Could you check a few things on this model? Use its own coordinates, in mm. A direction names the side the tool comes from. Round coordinates to 2 decimals unless told otherwise and drop trailing zeros. Loops run counter-clockwise (first coordinate to the right, second up) from the corner with the lowest first, then second, coordinate; pieces in that order, holes last.
from build123d import *

# Parameters (mm, degrees)
F2_R     = 7.5
F2_R_2   = 5.5
F3_DEPTH = 3
F4_DEPTH = 5


# Not quite as in the source:
# - a feature names something its author has since deleted; it is built from what else it names


with BuildPart() as f3:
    # F2 (on Top) → F3 (new body)
    with BuildSketch(Plane.XY):
        with BuildLine():
            Line((120, 9.5), (0, 9.5))
            ThreePointArc((0, 9.5), (-6.7175144213, 6.7175144213), (-9.5, 0))
            ThreePointArc((-9.5, 0), (-6.7175144213, -6.7175144213), (0, -9.5))
            Line((0, -9.5), (120, -9.5))
            ThreePointArc((120, -9.5), (126.7175144213, -6.7175144213), (129.5, 0))
            ThreePointArc((129.5, 0), (126.7175144213, 6.7175144213), (120, 9.5))
        make_face()
        Circle(F2_R, mode=Mode.SUBTRACT)
        with Locations((20, 0)):
            Circle(F2_R, mode=Mode.SUBTRACT)
        with Locations((40, 0)):
            Circle(F2_R, mode=Mode.SUBTRACT)
        with Locations((60, 0)):
            Circle(F2_R, mode=Mode.SUBTRACT)
        with Locations((80, 0)):
            Circle(F2_R, mode=Mode.SUBTRACT)
        with Locations((100, 0)):
            Circle(F2_R, mode=Mode.SUBTRACT)
        with Locations((120, 0)):
            Circle(F2_R, mode=Mode.SUBTRACT)
        Circle(F2_R)
        Circle(F2_R_2, mode=Mode.SUBTRACT)
        with Locations((20, 0)):
            Circle(F2_R)
        with Locations((20, 0)):
            Circle(F2_R_2, mode=Mode.SUBTRACT)
        with Locations((40, 0)):
            Circle(F2_R)
        with Locations((40, 0)):
            Circle(F2_R_2, mode=Mode.SUBTRACT)
        with Locations((60, 0)):
            Circle(F2_R)
        with Locations((60, 0)):
            Circle(F2_R_2, mode=Mode.SUBTRACT)
        with Locations((80, 0)):
            Circle(F2_R)
        with Locations((80, 0)):
            Circle(F2_R_2, mode=Mode.SUBTRACT)
        with Locations((100, 0)):
            Circle(F2_R)
        with Locations((100, 0)):
            Circle(F2_R_2, mode=Mode.SUBTRACT)
        with Locations((120, 0)):
            Circle(F2_R)
        with Locations((120, 0)):
            Circle(F2_R_2, mode=Mode.SUBTRACT)
    extrude(amount=F3_DEPTH)

    # F2 (on Top) → F4 (join)
    with BuildSketch(Plane.XY):
        Circle(F2_R)
        Circle(F2_R_2, mode=Mode.SUBTRACT)
        with Locations((20, 0)):
            Circle(F2_R)
        with Locations((20, 0)):
            Circle(F2_R_2, mode=Mode.SUBTRACT)
        with Locations((40, 0)):
            Circle(F2_R)
        with Locations((40, 0)):
            Circle(F2_R_2, mode=Mode.SUBTRACT)
        with Locations((60, 0)):
            Circle(F2_R)
        with Locations((60, 0)):
            Circle(F2_R_2, mode=Mode.SUBTRACT)
        with Locations((80, 0)):
            Circle(F2_R)
        with Locations((80, 0)):
            Circle(F2_R_2, mode=Mode.SUBTRACT)
        with Locations((100, 0)):
            Circle(F2_R)
        with Locations((100, 0)):
            Circle(F2_R_2, mode=Mode.SUBTRACT)
        with Locations((120, 0)):
            Circle(F2_R)
        with Locations((120, 0)):
            Circle(F2_R_2, mode=Mode.SUBTRACT)
    extrude(amount=F4_DEPTH)


solid = f3.part
Item 1: We'd pull the mould along X, two halves only. Please class faces 3 (the cylindrical face through (12.507, 0.33, 3.986)), 4 (the flat face through (76, 4, 5)): released by +X, released by -X, zero draft, split by the parting line, or undercut.
Results list:
face 3: undercut
face 4: zero draft
Item 2: If I drill on line 1 along Y through (x, z) = (40, 2.4); line 2 along Z through (x, y) = (117.5, -7.75); line 3 along Y through (x, z) = (44.5, 2.75), over which ranges is the centre line in solid material (lowest first)?
Results list:
line 1: y = -9.5 to -5.5, 5.5 to 9.5
line 2: z = 0 to 3
line 3: y = -9.5 to -3.16, 3.16 to 9.5
Item 3: If we section it at A-A, the plane x = 80: Please give me the cut outline in (y, z).
Results list:
outline: (-9.5, 0) - (-5.5, 0) - (-5.5, 5) - (-7.5, 5) - (-7.5, 3) - (-9.5, 3) - close; (5.5, 0) - (9.5, 0) - (9.5, 3) - (7.5, 3) - (7.5, 5) - (5.5, 5) - close
Item 4: If we section it at C-C, the plane x = 104: Please give me the cut outline in (y, z), then the cut area to 3 significant figures.
Results list:
outline: (-9.5, 0) - (-3.77, 0) - (-3.77, 5) - (-6.34, 5) - (-6.34, 3) - (-9.5, 3) - close; (3.77, 0) - (9.5, 0) - (9.5, 3) - (6.34, 3) - (6.34, 5) - (3.77, 5) - close
area: 44.6 mm2
Item 5: If we section it at B-B, the plane z = 2: Please give me the cut outline in (x, y), then the cut area to 3 significant figures.
Results list:
outline: (0, -9.5) - (120, -9.5) arc R9.5 ccw to (120, 9.5) - (0, 9.5) arc R9.5 ccw to start; hole circle Ø11 at (0, 0); hole circle Ø11 at (20, 0); hole circle Ø11 at (40, 0); hole circle Ø11 at (60, 0); hole circle Ø11 at (80, 0); hole circle Ø11 at (100, 0); hole circle Ø11 at (120, 0)
area: 1,900 mm2
Item 6: If we section it at D-D, the plane y = 1.25: Count the separate pieces of the cut face and the enclosed holes in it, then the cut area to 3 significant figures.
Results list:
separate pieces: 8
enclosed holes: 0
area: 249 mm2
Item 7: For faces 1 (the flat face through (16, 4, 5)), 2 (the flat face through (59, -8, 3)), which set-ups out of +Z, -Z, +X, -X, +Y, -Y let a thin tool reach every point of the face, with its end or its side?
Results list:
face 1: +Z, +X, -X, +Y, -Y
face 2: +Z
